Answer from the drawing. Dimensions are ordinates in mm from the lowest x, y and z of the part. Give positions to 0.01 mm unless a question says otherwise; leave off trailing zeros. Order: outer loops, then holes, each group sorted by start corner. A loop starts at its lowest first (then second) coordinate and runs counter-clockwise, first axis right, second up. Notation, with made-up numbers: (35.5, 72.5) -> (64.5, 72.5) arc R19 cw to (64.5, 88.5) -> close; hole circle Ø2 at (78, 78.25). An arc over 180 degrees is marked (long way). Answer as CSV lines item,"result". Start each with the question number.
1) The mould has two halves that part along X. Classify the marked faces 1, 2, 3 and 4: +X half, -X half, draft (parallel to the pull), parting line (faces both ways), or undercut.
2) Find section D-D (x = 86). Determine the outline of the cut face in (y, z), and give its area (3 significant figures).
3) Straight lines are drawn through the part: L1, parallel to X at y = 44, z = 14 (1 decimal); L2, parallel to Y at x = 47.5, z = 13.5 (1 decimal); L3, parallel to Y at x = 29.5, z = 14 (1 decimal). For each, find the intervals that lie inside material, in ascending order. Write a range as from..to.
4) Flat-ended cylindrical pins translate along their axes: pin 1 Ø4 at (x, z) = (56, 6.5) entering from +Y; pin 2 Ø3 at (x, y) = (29.5, 61) entering from -Z; pin 3 Ø4 at (y, z) = (54, 11) entering from +X; pin 4 Ø6 at (x, z) = (85.5, 15.5) entering from -Y. Find the tip coordinate at first contact, or state that the pin passes through.
5) Find section B-B (y = 10). Determine the outline of the cut face in (x, z), and give its area (3 significant figures).
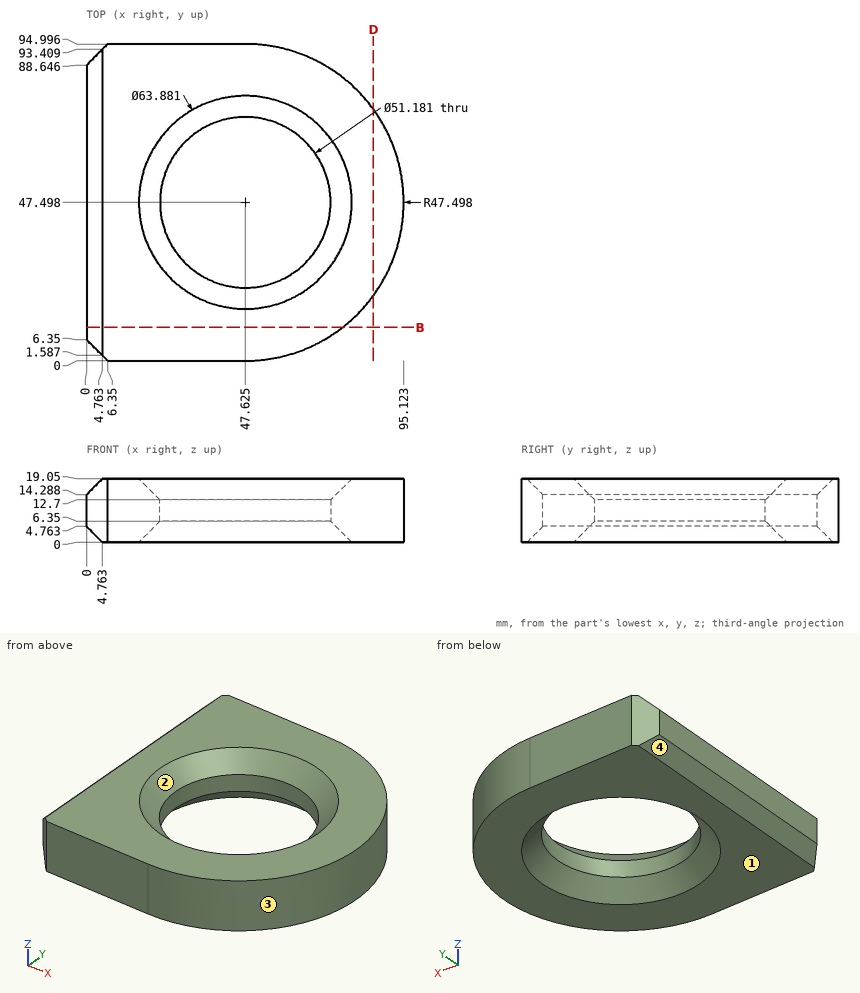
Findings below:
1,face 1,"draft"
1,face 2,"undercut"
1,face 3,"+X half"
1,face 4,"-X half"
2,outline,"(19.51, 0) -> (75.49, 0) -> (75.49, 19.05) -> (19.51, 19.05) -> close"
2,area,"1,070 mm²"
3,L1,"0..21, 74.3..95"
3,L2,"0..21.1, 73.9..95"
3,L3,"0..27.6, 67.4..95"
4,pin 1,"y = 94.57"
4,pin 2,"through"
4,pin 3,"x = 94.91"
4,pin 4,"y = 15.25"
5,outline,"(0, 4.76) -> (4.76, 0) -> (76.78, 0) -> (76.78, 19.05) -> (4.76, 19.05) -> (0, 14.29) -> close"
5,area,"1,440 mm²"
